Check sheet for the drawn part. Datum: minimum x, y, z corner. Units: mm. A direction names the side the tool comes from. Coordinates: 2 decimals unless noted, no trailing zeros. Order: outer loops, then holes, each group sorted by start corner. A loop starts at its lowest first (then second) coordinate and runs counter-clockwise, first axis right, second up. Notation, with made-up numbers: (25, -12.75) - (66, -12.75) arc R7 cw to (66, -0.75) - close; hole circle Ø5 at (75.25, 15). An arc over 180 degrees is marked (long way). One line per item, written item: value. Start each with the question number.
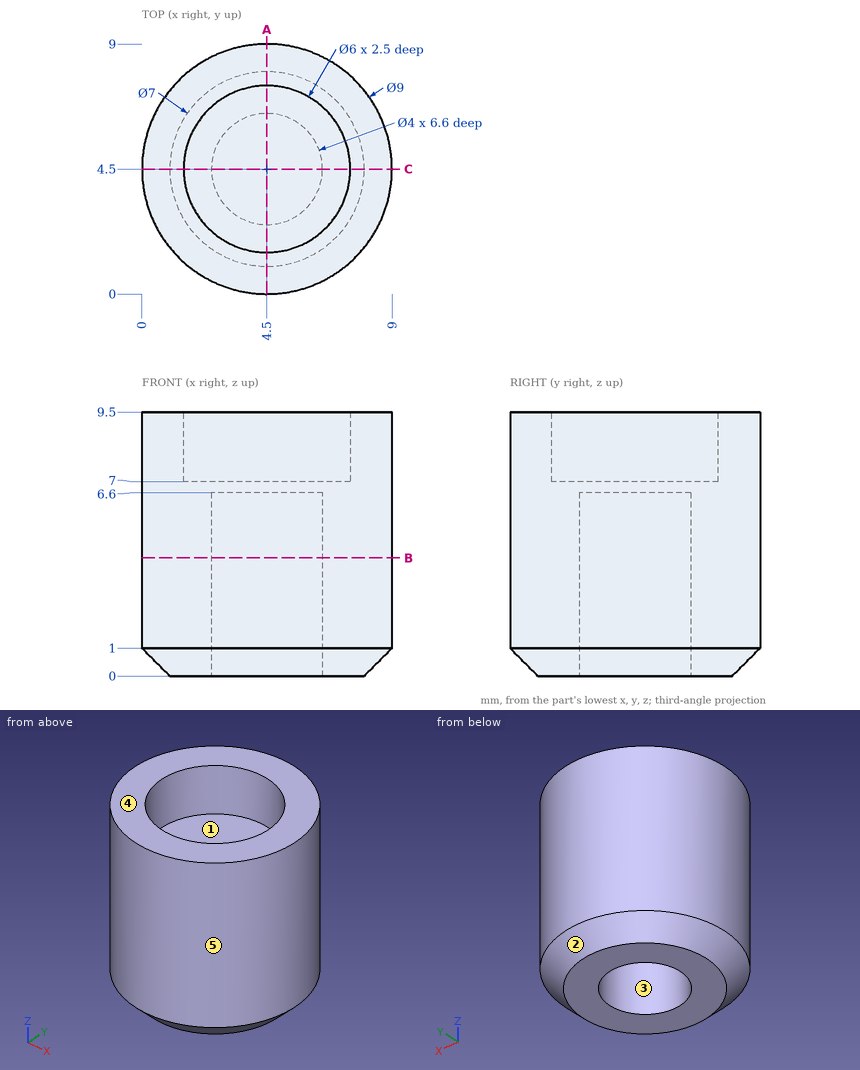
Q1. Material ranges on probe 1 along Y at (x, z) = (4.5, 8.4); probe 2 along Z at (x, y) = (7, 4.5); probe 3 along X at (y, z) = (2.5, 8.5), recorded low to high.
Q2. Gauge pin test, flat ends, axial feed: P1, Ø3, axis at x = 5, y = 3.5, coming from the +Z side; P2, Ø1.2, axis at x = 5.5, y = 4, coming from the -Z side; P3, Ø5, axis at x = 7.5, z = 8, coming from the +Y side. Record the tip position at first contact, or that the pin passes through.
Q3. Release check for a two-part mould opening along X. For the marked faces 3, 4 and 5 record: released by +X, released by -X, zero draft, split by the parting line, or undercut.
Q4. Set-up check for the marked faces 1 and 2: record each of +Z, -Z, +X, -X, +Y, -Y from which the full face is reachable in a straight line by a thin tool's end or side.
Q5. Cross-section at B-B, the plane z = 4.25. Enter the section's corners in (x, y), and give its area (3 significant figures).
Q6. Cross-section at A-A, the plane x = 4.5. Enter the section's corners in (y, z), and give its area (3 significant figures).
Check result:
1. probe 1: y = 0 to 1.5, 7.5 to 9
1. probe 2: z = 0 to 7
1. probe 3: x = 0.47 to 2.26, 6.74 to 8.53
2. P1: stops at z = 7
2. P2: stops at z = 6.6
2. P3: stops at y = 8.97
3. face 3: undercut
3. face 4: zero draft
3. face 5: split by the parting line
4. face 1: +Z
4. face 2: -Z
5. outline: circle Ø9 at (4.5, 4.5); hole circle Ø4 at (4.5, 4.5)
5. area: 51.1 mm2
6. outline: (0, 1) - (1, 0) - (2.5, 0) - (2.5, 6.6) - (6.5, 6.6) - (6.5, 0) - (8, 0) - (9, 1) - (9, 9.5) - (7.5, 9.5) - (7.5, 7) - (1.5, 7) - (1.5, 9.5) - (0, 9.5) - close
6. area: 43.1 mm2
